Here's the drawing with two shaded views (mm, measured from the low corner). I have some questions. A direction names the side the tool comes from. Give positions to 0.01 mm unless a question says otherwise; leave off trailing zeros. Loops run counter-clockwise (first coordinate to the right, second up) from the corner with the lowest first, then second, coordinate; pieces in that order, holes last. Notation, with made-up numbers: (-19.75, -38.75) -> (29.25, -38.75) arc R18 cw to (29.25, -9.75) -> close; hole circle Ø2 at (-26.5, 70.25). An arc over 180 degrees is marked (long way). Write each question's results on one line, items separated by ' | '. Start each with the question number.
Q1. If we section it at B-B, the plane y = 17.5: List the corners of the cut face in (x, z) for me.
Q2. Will this pin go through, and if not, where does the flat tip stop? P1, Ø4, axis at x = 7, z = 5.5, coming from the -Y side.
Q3. If we section it at D-D, the plane x = 15.25: List the corners of the cut face in (y, z) for me.
Q4. If we section it at C-C, the plane z = 12: List the corners of the cut face in (x, y) for me, plus the area to 3 significant figures.
Q5. If I drill on line 1 along X through (y, z) = (9.25, 1); line 2 along Y through (x, z) = (5, 2); line 3 along Y through (x, z) = (7.5, 13.75) (1 decimal), over which ranges is the centre line in solid material (lowest first)?
Q6. Which directions (+Z, -Z, +X, -X, +Y, -Y) give clear straight access to the entire face, cutting with the end or side of a thin tool? Please do the marked faces 1 and 2.
Q7. We'd pull the mould along X, two halves only. Please class the marked faces 3, 4, 5 and 6: released by +X, released by -X, zero draft, split by the parting line, or undercut.
Q8. If we section it at A-A, the plane x = 2.5: List the corners of the cut face in (y, z) for me.
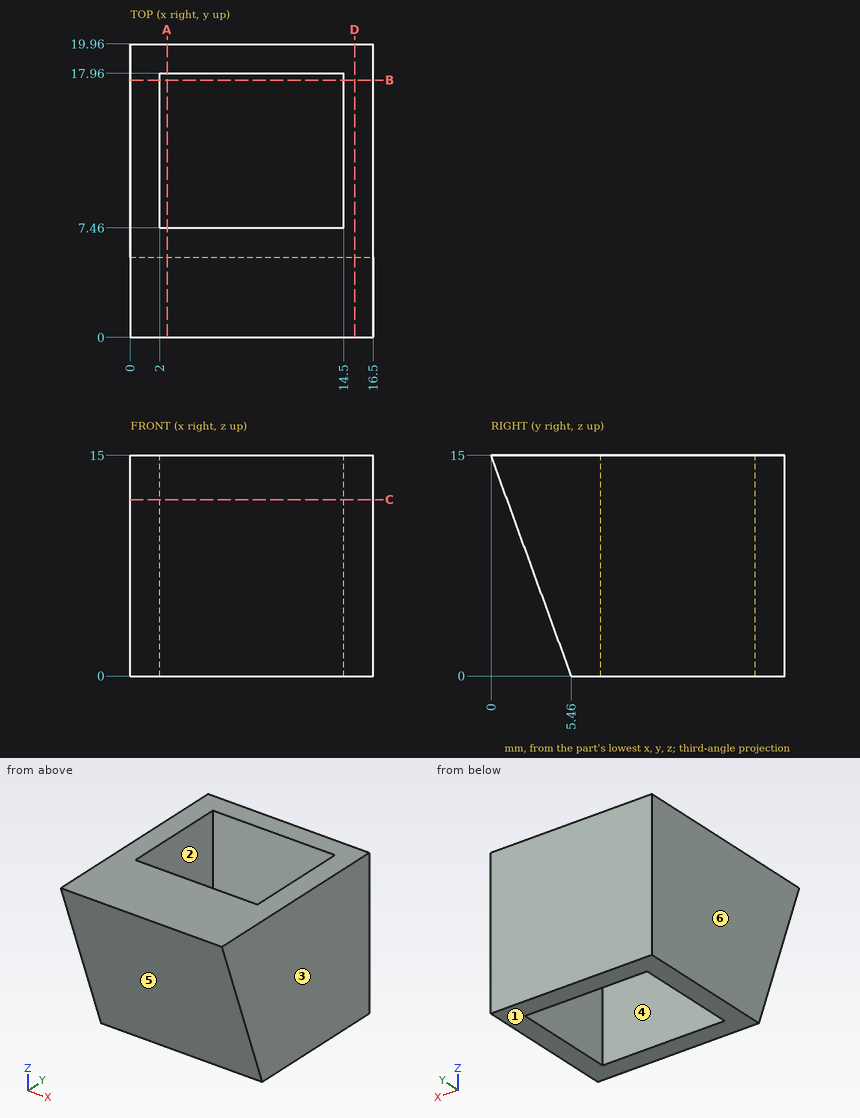
Final values:
1) outline: (0, 0) -> (2, 0) -> (2, 15) -> (0, 15) -> close; (14.5, 0) -> (16.5, 0) -> (16.5, 15) -> (14.5, 15) -> close
2) P1: stops at y = 2.73
3) outline: (0, 15) -> (5.46, 0) -> (19.96, 0) -> (19.96, 15) -> close
4) outline: (0, 1.09) -> (16.5, 1.09) -> (16.5, 19.96) -> (0, 19.96) -> close; hole (2, 7.46) -> (14.5, 7.46) -> (14.5, 17.96) -> (2, 17.96) -> close | area: 180 mm²
5) line 1: x = 0 to 2, 14.5 to 16.5 | line 2: y = 4.73 to 7.46, 17.96 to 19.96 | line 3: y = 0.5 to 7.5, 18 to 20
6) face 1: -Z, +X, -X, +Y, -Y | face 2: +Z, -Z
7) face 3: released by +X | face 4: undercut | face 5: zero draft | face 6: released by -X
8) outline: (0, 15) -> (5.46, 0) -> (7.46, 0) -> (7.46, 15) -> close; (17.96, 0) -> (19.96, 0) -> (19.96, 15) -> (17.96, 15) -> close
